from build123d import *


with BuildPart() as part:
    # Sketch1 → Revolve1 (revolve)
    with BuildSketch(Plane.XY, mode=Mode.PRIVATE) as revolve1_sk:
        with BuildLine():
            Line((12.192, -3.17754), (12.192, -3.14579))
            ThreePointArc((12.192, -3.14579), (12.415184633, -2.606974633), (12.954, -2.38379))
            Line((12.954, -2.38379), (16.764, -2.38379))
            Line((16.764, -2.38379), (17.78, -1.910021419))
            Line((17.78, -1.910021419), (17.78, 0))
            Line((17.78, 0), (8.89, 0))
            Line((8.89, 0), (0, 0))
            Line((0, 0), (0, -2.921))
            Line((0, -2.921), (1.454910638, -3.17754))
            Line((1.454910638, -3.17754), (12.192, -3.17754))
        make_face()
    revolve(revolve1_sk.sketch.rotate(Axis((0, 0, 0), (-1, 0, 0)), 180), axis=Axis((0, 0, 0), (-1, 0, 0)))  # turned: the seam where the file's is


solid = part.part
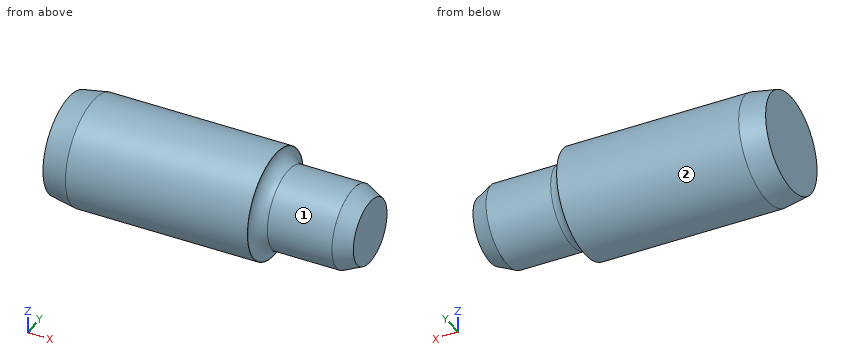
Design review of the part built by this model. Coordinates are the model's own, in mm. Face numbers are marked on the shaded views. A direction names the side the tool comes from. Give positions to 0.01 mm unless a question says otherwise; leave off trailing zeros. Order: outer loops, then holes, each group sorted by start corner. A loop starts at its lowest first (then second) coordinate and runs counter-clockwise, first axis right, second up. Notation, with made-up numbers: (85, 49) - (110, 49) arc R20 cw to (110, 77) - close; hole circle Ø4 at (66.25, -35). An arc over 180 degrees is marked (long way). Write item = value, one per line. Start each with the question number.
Q1. We need section C-C on x = 3. State the section outline as (y, z) points, plus the area to 3 significant figures.
Q2. Tool access review of the marked faces 1 and 2: name each direction out of +Z, -Z, +X, -X, +Y, -Y from which nothing blocks a thin tool from reaching the whole face with its end or side.
Q3. To check wall thickness, follow L1, parallel to Z at x = 14, y = 0; L2, parallel to Y at x = 13.5, z = 1.5; L3, parallel to Y at x = 9.25, z = -0.75. State the ranges of each line that lie inside material, in increasing order. Write a range as from..to.
Q4. Clearance check with flat-ended pins moving along their axes: pin 1 Ø1 at (x, z) = (7, -1.5) entering from -Y; pin 2 Ø2 at (x, z) = (9, -1.5) entering from +Y; pin 3 Ø1.5 at (x, y) = (8, 1.5) entering from -Z. State where each tip first meets the part, or that it passes through.
Working result:
q1.outline = circle Ø6.36 at (0, 0)
q1.area = 31.7 mm²
q2.face_1 = +X
q2.face_2 = +X, -X
q3.L1 = -2.38..2.38
q3.L2 = -1.85..1.85
q3.L3 = -3.09..3.09
q4.pin_1 = -3.02
q4.pin_2 = 3.14
q4.pin_3 = -3.09
